The listing builds one solid part. Answer for the finished solid, in the listing's coordinates (mm). Round coordinates to 2 decimals unless told otherwise and drop trailing zeros. Write each loop counter-clockwise with the first axis right and the second up, starting at its lowest first coordinate (ties: lowest second). Pieces come first, ordered by that corner, then holes.
Item 1: Find section C-C on x = 3. Give the vertices of the cut face in (y, z).
Item 2: Find the intervals of material crossed by probe 1 along Y at (x, z) = (-3, 4.5); probe 2 along Y at (x, z) = (-6, 0.5); probe 3 along X at (y, z) = (-5, 6), in increasing order.
Item 3: Each of these flat-tipped pins is pushed along its axis until it touches: pin 1 (3 mm diameter, centred on x = -4.72, y = -2.09, fed in from -Z); pin 2 (1.5 mm diameter, centred on y = 0.5, z = 1.5, fed in from -X). Where does it stop, or does it pass through?
Item 4: For a pull along X with two mould halves and no side action, classify faces 1 (the face through (-55.117, -1.984, 3.885)), 2 (the face through (-71.21, -4.73, 3.88)), 3 (the face through (13.77, 0.55, 3.88)), 4 (the face through (-28, 1.606, 4)) as +X half, -X half, draft (parallel to the pull), parting line (faces both ways), or undercut.
Item 5: Find section B-B on z = 5.25. Give the number of separate pieces and of enclosed holes in the cut face, then the cut area to 3 significant figures.
Item 6: Find section A-A on x = -14. Give the vertices of the cut face in (y, z), then the cut area to 3 significant figures.
```python
from build123d import *

# Parameters (mm, degrees)
F0_R        = 2.4
F1_DEPTH    = 7.88
F2_T1_DEPTH = 26.405


# Not quite as in the source:
# - a fillet or chamfer that OpenCascade refuses, or shapes differently, is made with other operations: its cross-section is extruded or revolved along the edge and cut away or added


with BuildPart() as f1:
    # F0 (on Top) → F1 (new body)
    with BuildSketch(Plane.XY):
        Polygon((14.8854916829, 1.6058013724), (-28.7195083171, 1.6058013724), (-72.3245083171, 1.6058013724), (-72.3245083171, -2.0891986276), (-72.3245083171, -5.7841986276), (-28.7195083171, -5.7841986276), (14.8854916829, -5.7841986276), (14.8854916829, -2.0891986276), align=None)
        with Locations((-68.7195083171, -2.0891986276)):
            Circle(F0_R, mode=Mode.SUBTRACT)
        with Locations((-60.7195083171, -2.0891986276)):
            Circle(F0_R, mode=Mode.SUBTRACT)
        with Locations((-52.7195083171, -2.0891986276)):
            Circle(F0_R, mode=Mode.SUBTRACT)
        with Locations((-44.7195083171, -2.0891986276)):
            Circle(F0_R, mode=Mode.SUBTRACT)
        with Locations((-36.7195083171, -2.0891986276)):
            Circle(F0_R, mode=Mode.SUBTRACT)
        with BuildLine():
            ThreePointArc((-28.7195083171, -4.4891986276), (-31.1195083171, -2.0891986276), (-28.7195083171, 0.3108013724))
            ThreePointArc((-28.7195083171, 0.3108013724), (-26.3195083171, -2.0891986276), (-28.7195083171, -4.4891986276))
        make_face(mode=Mode.SUBTRACT)
        with Locations((-20.7195083171, -2.0891986276)):
            Circle(F0_R, mode=Mode.SUBTRACT)
        with Locations((-12.7195083171, -2.0891986276)):
            Circle(F0_R, mode=Mode.SUBTRACT)
        with Locations((-4.7195083171, -2.0891986276)):
            Circle(F0_R, mode=Mode.SUBTRACT)
        with Locations((3.2804916829, -2.0891986276)):
            Circle(F0_R, mode=Mode.SUBTRACT)
        with Locations((11.2804916829, -2.0891986276)):
            Circle(F0_R, mode=Mode.SUBTRACT)
    extrude(amount=F1_DEPTH)

    # F2: fillet of radius 3.705 on 4 edges, made by hand

    # F2_s2 → F2_t1 (cut)
    with BuildSketch(Plane.XY.offset(-9.2625)):
        with BuildLine():
            ThreePointArc((11.1804916829, 1.6058013724), (13.8003223072, 0.5206319967), (14.8854916829, -2.0991986276))
            Line((14.8854916829, -2.0991986276), (14.8854916829, 1.6058013724))
            Line((14.8854916829, 1.6058013724), (11.1804916829, 1.6058013724))
        make_face()
        with BuildLine():
            ThreePointArc((11.1804916829, -5.7841986276), (13.8003223072, -4.6990292519), (14.8854916829, -2.0791986276))
            Line((14.8854916829, -2.0791986276), (14.8854916829, -5.7841986276))
            Line((14.8854916829, -5.7841986276), (11.1804916829, -5.7841986276))
        make_face()
        with BuildLine():
            ThreePointArc((-68.6195083171, 1.6058013724), (-71.2393389413, 0.5206319967), (-72.3245083171, -2.0991986276))
            Line((-72.3245083171, -2.0991986276), (-72.3245083171, 1.6058013724))
            Line((-72.3245083171, 1.6058013724), (-68.6195083171, 1.6058013724))
        make_face()
        with BuildLine():
            ThreePointArc((-68.6195083171, -5.7841986276), (-71.2393389413, -4.6990292519), (-72.3245083171, -2.0791986276))
            Line((-72.3245083171, -2.0791986276), (-72.3245083171, -5.7841986276))
            Line((-72.3245083171, -5.7841986276), (-68.6195083171, -5.7841986276))
        make_face()
    extrude(amount=F2_T1_DEPTH, mode=Mode.SUBTRACT)


solid = f1.part
```
Check values:
1. outline: (-5.78, 0) - (-4.47, 0) - (-4.47, 7.88) - (-5.78, 7.88) - close; (0.29, 0) - (1.61, 0) - (1.61, 7.88) - (0.29, 7.88) - close
2. probe 1: y = -5.78 to -3.76, -0.41 to 1.61
2. probe 2: y = -5.78 to -4.12, -0.06 to 1.61
2. probe 3: x = -70.9 to 13.46
3. pin 1: passes through
3. pin 2: stops at x = -71.83
4. face 1: undercut
4. face 2: -X half
4. face 3: +X half
4. face 4: draft
5. separate pieces: 1
5. enclosed holes: 11
5. area: 434 mm2
6. outline: (-5.78, 0) - (-4.12, 0) - (-4.12, 7.88) - (-5.78, 7.88) - close; (-0.06, 0) - (1.61, 0) - (1.61, 7.88) - (-0.06, 7.88) - close
6. area: 26.2 mm2
